```python
from build123d import *

# Parameters (mm, degrees)
ESQUISSE1_W           = 6
ESQUISSE1_H           = 6
BOSS_EXTRU_2_DEPTH    = 3.5
BOSS_EXTRU_3_DEPTH    = 1.2
CONG_2_R              = 1.2
CONG_2_OF_SYM_TRIE2_R = 1.2


with BuildPart() as part:
    # Esquisse1 → Boss.-Extru.2 (new body)
    with BuildSketch(Plane(origin=(0, 0, 0), x_dir=(1, 0, 0), z_dir=(0, 1, 0))):
        with BuildLine():
            ThreePointArc((19.364916731, -35), (0, 40), (-19.364916731, -35))
            ThreePointArc((-19.364916731, -35), (-9.581446139, -30.851796587), (-13.564659966, -21))
            ThreePointArc((-13.564659966, -21), (0, 25), (13.564659966, -21))
            ThreePointArc((13.564659966, -21), (9.581446139, -30.851796587), (19.364916731, -35))
        make_face()
        with Locations((0, 32.5)):
            Rectangle(ESQUISSE1_W, ESQUISSE1_H, mode=Mode.SUBTRACT)
    extrude(amount=BOSS_EXTRU_2_DEPTH)

    # Esquisse5 → Boss.-Extru.3 (add)
    with BuildSketch(Plane(origin=(0, 3.5, 0), x_dir=(1, 0, 0), z_dir=(0, 1, 0))):
        with BuildLine():
            ThreePointArc((-20.075175272, -28.67032155), (-34.468271355, 6.077686218), (-9.058666579, 33.80740392))
            ThreePointArc((-9.058666579, 33.80740392), (-6.915363054, 32.569967053), (-8.152799921, 30.426663528))
            ThreePointArc((-8.152799921, 30.426663528), (-31.02144422, 5.469917597), (-18.067657745, -25.803289395))
            ThreePointArc((-18.067657745, -25.803289395), (-17.637900431, -28.240564236), (-20.075175272, -28.67032155))
        make_face()
    boss_extru_3 = extrude(amount=BOSS_EXTRU_3_DEPTH)

    # Congé2
    cong_2_edges = [part.edges().sort_by_distance(p)[0] for p in [
        (-34.468271355, 4.7, -6.077686218),
        (-6.915363054, 4.7, -32.569967053),
        (-31.02144422, 4.7, -5.469917597),
        (-17.637900431, 4.7, 28.240564236),
    ]]
    fillet(cong_2_edges, radius=CONG_2_R - 0.0001)  # a hair under: the kernel refuses the full size

    # Symétrie2: Boss.-Extru.3 across plane
    add(boss_extru_3.mirror(Plane(origin=(0, 0, 0), x_dir=(0, 0, 1), z_dir=(1, 0, 0))))

    # Congé2 of Symétrie2
    cong_2_of_sym_trie2_edges = [part.edges().sort_by_distance(p)[0] for p in [
        (34.468271355, 4.7, -6.077686218),
        (6.915363054, 4.7, -32.569967053),
        (31.02144422, 4.7, -5.469917597),
        (17.637900431, 4.7, 28.240564236),
    ]]
    fillet(cong_2_of_sym_trie2_edges, radius=CONG_2_OF_SYM_TRIE2_R - 0.0001)  # a hair under: the kernel refuses the full size


solid = part.part
```
Model file for the job. Use its own axes, mm. A direction names the side the tool comes from. Coordinates: 2 decimals unless noted, no trailing zeros. Loops run counter-clockwise (first coordinate to the right, second up) from the corner with the lowest first, then second, coordinate; pieces in that order, holes last. Notation, with made-up numbers: (38.5, 44) - (61.5, 44) arc R25 ccw to (61.5, 62) - close; hole circle Ø8 at (17.25, -30.5). An arc over 180 degrees is marked (long way). Answer as a JSON object with one key per item and string values. Group by question number.
(1) Probe line 1 along X through (y, z) = (1.5, 0); line 2 along X through (y, z) = (0.55, -11.5); line 3 along Z through (x, y) = (17.5, 0.45). List the from-to ranges inside material, lowest first.
(2) Cut at A-A (x = 0). Give the cut face in (y, z), then the cut area to 3 significant figures.
(3) Flat gauge pins, fed straight in: pin 1 (2 mm diameter, centred on x = -6.5, y = 1.5, fed in from +Z); pin 2 (1 mm diameter, centred on y = 1, z = -24, fed in from +X); pin 3 (1 mm diameter, centred on x = -1, y = 1.5, fed in from -Z). Where does each tip first touch, or does it go through?
(4) Cut at B-B (y = 2). Give the cut face in (x, z), then the cut area to 3 significant figures.
(5) Tool access for faces 4 (the face through (-32.3, 4.7, -7.1)), 5 (the face through (-18, 3.5, -20)), 6 (the face through (3, 2, -32)): list every direction of +Z, -Z, +X, -X, +Y, -Y with a clear straight run to the whole face (end or side of a thin tool).
(6) Two-plate mould, pull along Z, no slides. Class faces 1 (the face through (1.476, 1.726, -39.973)), 2 (the face through (-3, 2, -32)), 3 (the face through (32.3, 4.7, -7.1)): released by +Z, released by -Z, zero draft, split by the parting line, or undercut.
Geometry says:
{
 "1": {"line 1": "x = -40 to -25, 25 to 40", "line 2": "x = -38.31 to -22.2, 22.2 to 38.31", "line 3": "z = -35.97 to -17.85, 17.85 to 35.47"},
 "2": {"outline": "(0, -40) - (3.5, -40) - (3.5, -35.5) - (0, -35.5) - close; (0, -29.5) - (3.5, -29.5) - (3.5, -25) - (0, -25) - close", "area": "31.5 mm^2"},
 "3": {"pin 1": "stops at z = -23.85", "pin 2": "stops at x = 32.37", "pin 3": "stops at z = -40"},
 "4": {"outline": "(-19.36, 35) arc R40 ccw (long way) to (19.36, 35) arc R7.58 ccw to (13.56, 21) arc R25 cw (long way) to (-13.56, 21) arc R7.58 ccw to start; hole (-3, -35.5) - (3, -35.5) - (3, -29.5) - (-3, -29.5) - close", "area": "2,690 mm^2"},
 "5": {"face 4": "+Z, -Z, +X, -X, +Y", "face 5": "+Y", "face 6": "+Y, -Y"},
 "6": {"face 1": "split by the parting line", "face 2": "undercut", "face 3": "zero draft"}
}
